from build123d import *

# Parameters (mm, degrees)
BOSS_EXTRUDE1_DEPTH = 0.05
FILLET1_R           = 1


with BuildPart() as part:
    # frame_outline → Boss-Extrude1 (new, symmetric)
    with BuildSketch(Plane.XY):
        Polygon((0.5, 0), (3, 0), (3, -0.25), (4, -0.25), (4, 0), (4.5, 0), (5.266044443, 0.64278761), (5.426741346, 0.451276499), (6.192785789, 1.094064109), (6.032088886, 1.285575219), (6.606622219, 1.767665927), (5.050898392, 1.767665927), (4.136029766, 1), (-4.136029766, 1), (-5.050898392, 1.767665927), (-6.606622219, 1.767665927), (-6.032088886, 1.285575219), (-6.192785789, 1.094064109), (-5.426741346, 0.451276499), (-5.266044443, 0.64278761), (-4.5, 0), (-4, 0), (-4, -0.25), (-3, -0.25), (-3, 0), (-0.5, 0), (-0.5, -0.25), (0.5, -0.25), align=None)
    extrude(amount=BOSS_EXTRUDE1_DEPTH, both=True)

    # Fillet1
    fillet1_edges = [part.edges().sort_by_distance(p)[0] for p in [
        (-5.050898392, 1.767665927, 0),
        (-4.136029766, 1, 0),
        (4.136029766, 1, 0),
        (5.050898392, 1.767665927, 0),
    ]]
    fillet(fillet1_edges, radius=FILLET1_R)


solid = part.part
The listing builds one solid part. Answer for the finished solid, in the listing's coordinates (mm). Give positions to 0.01 mm unless a question says otherwise; leave off trailing zeros. Loops run counter-clockwise (first coordinate to the right, second up) from the corner with the lowest first, then second, coordinate; pieces in that order, holes last.
Item 1: A cutting plane is placed at A-A (y = 1.4). Give the vertices of the cut face in (x, z), then the cut area to 3 significant figures.
Derived:
outline: (-6.17, -0.05) - (-4.61, -0.05) - (-4.61, 0.05) - (-6.17, 0.05) - close; (4.61, -0.05) - (6.17, -0.05) - (6.17, 0.05) - (4.61, 0.05) - close
area: 0.311 mm2
Item 2: A cutting plane is placed at B-B (x = 0.25). Give the vertices of the cut face in (y, z).
Derived:
outline: (-0.25, -0.05) - (1, -0.05) - (1, 0.05) - (-0.25, 0.05) - close
Item 3: Find the intervals of material crossed by line 1 along X through (y, z) = (0.55, 0); line 2 along X through (y, z) = (1.5, 0); line 3 along Y through (x, z) = (5, 0), in increasing order.
Derived:
line 1: x = -5.54 to -5.34, -5.16 to 5.16, 5.34 to 5.54
line 2: x = -6.29 to -4.73, 4.73 to 6.29
line 3: y = 0.42 to 1.68
Item 4: A cutting plane is placed at C-C (y = 0.3). Give the vertices of the cut face in (x, z).
Derived:
outline: (-4.86, -0.05) - (4.86, -0.05) - (4.86, 0.05) - (-4.86, 0.05) - close
